from build123d import *

# Parameters (mm, degrees)
SKETCH1_W           = 15
SKETCH1_H           = 30
SKETCH1_R           = 4
BOSS_EXTRUDE1_DEPTH = 5
SKETCH3_R           = 1.5
CUT_EXTRUDE1_DEPTH  = 30
SKETCH2_R           = 2.5
CUT_EXTRUDE2_DEPTH  = 10
FILLET1_R           = 3


with BuildPart() as part:
    # Sketch1 → Boss-Extrude1 (new body)
    with BuildSketch(Plane.XY):
        with Locations((0, 5)):
            Rectangle(SKETCH1_W, SKETCH1_H)
        Circle(SKETCH1_R, mode=Mode.SUBTRACT)
    extrude(amount=BOSS_EXTRUDE1_DEPTH)

    # Sketch3 → Cut-Extrude1 (cut)
    with BuildSketch(Plane(origin=(0, 0, 0), x_dir=(0, 0, -1), z_dir=(0, 1, 0))):
        with Locations(Location((-2.5, 0, 0), (0, 0, 180))):
            Circle(SKETCH3_R)
    extrude(amount=-CUT_EXTRUDE1_DEPTH, mode=Mode.SUBTRACT)

    # Sketch2 → Cut-Extrude2 (cut)
    with BuildSketch(Plane(origin=(0, -24.379216841, 5), x_dir=(1, 0, 0), z_dir=(0, 0, -1))):
        with Locations((0, -34.379216841)):
            Circle(SKETCH2_R)
    extrude(amount=CUT_EXTRUDE2_DEPTH, mode=Mode.SUBTRACT)

    # Fillet1
    fillet1_edges = [part.edges().sort_by_distance(p)[0] for p in [
        (-7.5, 20, 2.5),
        (7.5, 20, 2.5),
        (7.5, -10, 2.5),
        (-7.5, -10, 2.5),
    ]]
    fillet(fillet1_edges, radius=FILLET1_R)


solid = part.part
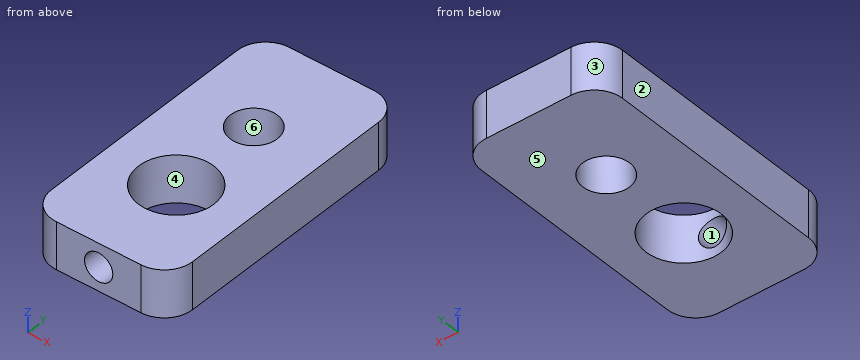
The model under review builds one solid part; all positions refer to its coordinate system, in mm. Face numbers are marked on the shaded views. A direction names the side the tool comes from. Round coordinates to 2 decimals unless told otherwise and drop trailing zeros. Loops run counter-clockwise (first coordinate to the right, second up) from the corner with the lowest first, then second, coordinate; pieces in that order, holes last. Notation, with made-up numbers: (21, 49) -> (78, 49) arc R20 cw to (78, 53) -> close; hole circle Ø7 at (17, 34.5). An arc over 180 degrees is marked (long way). Write item = value, one per line. Start each with the question number.
Item 1: Take a section at D-D on y = 0. Give the boundary of the cut face in (x, z).
Item 2: Take a section at C-C on z = 2.5. Give the boundary of the cut face in (x, y).
Item 3: Take a section at B-B on x = 0. Give the boundary of the cut face in (y, z).
Item 4: Mouldability with a two-part tool opening along X and no side actions: class the marked faces 3, 4, 5 and 6 as released by +X, released by -X, zero draft, split by the parting line, or undercut.
Item 5: For the marked faces 1 and 2, list the 3-axis set-ups (+Z, -Z, +X, -X, +Y, -Y) from which the entire face can be reached by the end or side of a thin tool; tool diameter is ignored.
Item 6: Take a section at A-A on y = 10. Give the boundary of the cut face in (x, z), plus the area to 3 significant figures.
Item 7: To check wall thickness, follow L1, parallel to X at y = 10, z = 2.9; L2, parallel to X at y = -5.75, z = 2.5; L3, parallel to Z at x = 0, y = -6. State the ranges of each line that lie inside material, in increasing order.
Result:
q1.outline = (-7.5, 0) -> (-4, 0) -> (-4, 5) -> (-7.5, 5) -> close; (4, 0) -> (7.5, 0) -> (7.5, 5) -> (4, 5) -> close
q2.outline = (-7.5, -7) arc R3 ccw to (-4.5, -10) -> (-1.5, -10) -> (-1.5, -3.71) arc R4 cw (long way) to (1.5, -3.71) -> (1.5, -10) -> (4.5, -10) arc R3 ccw to (7.5, -7) -> (7.5, 17) arc R3 ccw to (4.5, 20) -> (-4.5, 20) arc R3 ccw to (-7.5, 17) -> close; hole circle Ø5 at (0, 10)
q3.outline = (-10, 0) -> (-4, 0) -> (-4, 1) -> (-10, 1) -> close; (-10, 4) -> (-4, 4) -> (-4, 5) -> (-10, 5) -> close; (4, 0) -> (7.5, 0) -> (7.5, 5) -> (4, 5) -> close; (12.5, 0) -> (20, 0) -> (20, 5) -> (12.5, 5) -> close
q4.face_3 = released by -X
q4.face_4 = undercut
q4.face_5 = zero draft
q4.face_6 = undercut
q5.face_1 = -Y
q5.face_2 = +Z, -Z, -X, +Y, -Y
q6.outline = (-7.5, 0) -> (-2.5, 0) -> (-2.5, 5) -> (-7.5, 5) -> close; (2.5, 0) -> (7.5, 0) -> (7.5, 5) -> (2.5, 5) -> close
q6.area = 50.0 mm²
q7.L1 = -7.5 to -2.5, 2.5 to 7.5
q7.L2 = -7.5 to -1.5, 1.5 to 7.5
q7.L3 = 0 to 1, 4 to 5
